Check sheet for the modelled part. Datum: model origin and axes. Units: mm. Round coordinates to 2 decimals unless told otherwise and drop trailing zeros. Write each loop counter-clockwise with the first axis right and the second up, starting at its lowest first coordinate (ties: lowest second). Pieces come first, ordered by that corner, then holes. Notation, with made-up numbers: M 0,20.5 L 29,20.5 A17 ccw 29,25.5 Z; hole C 50.25,55.25 d7. An arc over 180 degrees is marked long. One line per item, written item: value.
from build123d import *

# Parameters (mm, degrees)
F0_R     = 2.5
F0_R_2   = 5
F0_R_3   = 4
F1_DEPTH = 1.5


with BuildPart() as f1:
    # F0 (on Top) → F1 (new body, symmetric)
    with BuildSketch(Plane.XY):
        Polygon((29, 55), (-29, 55), (-29, 45), (-34, 45), (-34, 25), (-29, 25), (-29, -25), (-34, -25), (-34, -45), (-29, -45), (-29, -55), (29, -55), (29, -45), (34, -45), (34, -25), (29, -25), (29, 25), (34, 25), (34, 45), (29, 45), align=None)
        with Locations((-10, 45)):
            Circle(F0_R, mode=Mode.SUBTRACT)
        with Locations((0, 30)):
            Circle(F0_R_2, mode=Mode.SUBTRACT)
        with Locations((10, 45)):
            Circle(F0_R_3, mode=Mode.SUBTRACT)
    extrude(amount=F1_DEPTH, both=True)


solid = f1.part
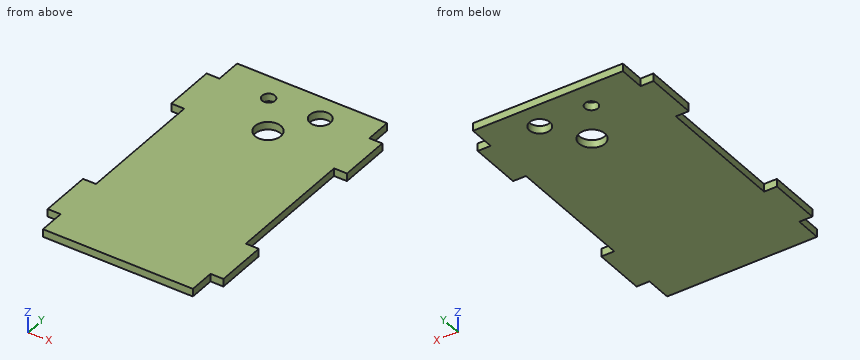
Q1. Sectioned sample at C-C on y = 31.5. Enter the section's corners in (x, z), and give its area (3 significant figures).
Completed:
outline: M -34,-1.5 L -4.77,-1.5 L -4.77,1.5 L -34,1.5 Z; M 4.77,-1.5 L 34,-1.5 L 34,1.5 L 4.77,1.5 Z
area: 175 mm^2
Q2. Sectioned sample at A-A on x = 0. Enter the section's corners in (y, z), and give its area (3 significant figures).
Completed:
outline: M -55,-1.5 L 25,-1.5 L 25,1.5 L -55,1.5 Z; M 35,-1.5 L 55,-1.5 L 55,1.5 L 35,1.5 Z
area: 300 mm^2
Q3. Sectioned sample at D-D on y = -9.5. Enter the section's corners in (x, z).
Completed:
outline: M -29,-1.5 L 29,-1.5 L 29,1.5 L -29,1.5 Z
Q4. Sectioned sample at B-B on z = -0.95. Enter the section's corners in (x, y).
Completed:
outline: M -34,-45 L -29,-45 L -29,-55 L 29,-55 L 29,-45 L 34,-45 L 34,-25 L 29,-25 L 29,25 L 34,25 L 34,45 L 29,45 L 29,55 L -29,55 L -29,45 L -34,45 L -34,25 L -29,25 L -29,-25 L -34,-25 Z; hole C -10,45 d5; hole C 0,30 d10; hole C 10,45 d8
Q5. Depth check by flat-ended pin: P1, Ø0.9, axis at x = -31.5, z = 0, coming from the +Y side; P2, Ø1.5, axis at y = -0.5, z = -0.5, coming from the -X side; P3, Ø0.9, axis at x = 30.5, z = -0.5, coming from the -Y side. Enter the tip coordinate at first touch or a pass-through.
Completed:
P1: y = 45
P2: x = -29
P3: y = -45
Q6. Scan lines: line 1 (Y direction, x = -10, z = -0.3); line 2 (Y direction, x = 0, z = -0.2); line 3 (X direction, y = 16, z = 0.2). Record each from-to range of solid material in increasing order. Write a range as [from, to].
Completed:
line 1: [-55, 42.5], [47.5, 55]
line 2: [-55, 25], [35, 55]
line 3: [-29, 29]
